Geometry check sheet. Reference: the model listing, model coordinates, mm. A direction names the side the tool comes from. Coordinates: 2 decimals unless noted, no trailing zeros. Write each loop counter-clockwise with the first axis right and the second up, starting at its lowest first coordinate (ties: lowest second). Pieces come first, ordered by that corner, then holes. Notation, with made-up numbers: (32.5, -10.5) -> (67.5, -10.5) arc R13 cw to (67.5, -4.5) -> close; hole circle Ø1 at (-26, -0.5). An arc over 180 degrees is marked (long way). Use a Markdown table: item, result.
```python
from build123d import *

# Parameters (mm, degrees)
SKETCH1_R           = 1.5
BOSS_EXTRUDE1_DEPTH = 25
SKETCH2_R           = 20
CUT_EXTRUDE1_DEPTH  = 23
CUT_EXTRUDE2_START  = -20
SKETCH3_R           = 1.5
CUT_EXTRUDE2_DEPTH  = 20
FILLET2_R           = 3
SKETCH4_R           = 22.5
SKETCH4_R_2         = 20
CUT_EXTRUDE3_DEPTH  = 2
CUT_EXTRUDE4_START  = -15
SKETCH5_R           = 24
CUT_EXTRUDE4_DEPTH  = 15
SKETCH6_R           = 22
CUT_EXTRUDE5_DEPTH  = 5


with BuildPart() as part:
    # Sketch1 → Boss-Extrude1 (new body)
    with BuildSketch(Plane(origin=(0, 0, 0), x_dir=(1, 0, 0), z_dir=(0, 1, 0))):
        with BuildLine():
            Line((13.169048105, 24), (-13.169048105, 24))
            Line((-13.169048105, 24), (-23.169048105, 26.882623622))
            ThreePointArc((-23.169048105, 26.882623622), (-26.121320344, 26.121320344), (-26.882623622, 23.169048105))
            Line((-26.882623622, 23.169048105), (-24, 13.169048105))
            Line((-24, 13.169048105), (-24, -13.169048105))
            Line((-24, -13.169048105), (-26.882623622, -23.169048105))
            ThreePointArc((-26.882623622, -23.169048105), (-26.121320344, -26.121320344), (-23.169048105, -26.882623622))
            Line((-23.169048105, -26.882623622), (-13.169048105, -24))
            Line((-13.169048105, -24), (13.169048105, -24))
            Line((13.169048105, -24), (23.169048105, -26.882623622))
            ThreePointArc((23.169048105, -26.882623622), (26.121320344, -26.121320344), (26.882623622, -23.169048105))
            Line((26.882623622, -23.169048105), (24, -13.169048105))
            Line((24, -13.169048105), (24, 13.169048105))
            Line((24, 13.169048105), (26.882623622, 23.169048105))
            ThreePointArc((26.882623622, 23.169048105), (26.121320344, 26.121320344), (23.169048105, 26.882623622))
            Line((23.169048105, 26.882623622), (13.169048105, 24))
        make_face()
        with Locations(Location((24, 24, 0), (0, 0, 270))):
            Circle(SKETCH1_R, mode=Mode.SUBTRACT)
        with Locations(Location((-24, -24, 0), (0, 0, 270))):
            Circle(SKETCH1_R, mode=Mode.SUBTRACT)
        with Locations(Location((24, -24, 0), (0, 0, 270))):
            Circle(SKETCH1_R, mode=Mode.SUBTRACT)
        with Locations(Location((-24, 24, 0), (0, 0, 270))):
            Circle(SKETCH1_R, mode=Mode.SUBTRACT)
    extrude(amount=BOSS_EXTRUDE1_DEPTH)

    # Sketch2 → Cut-Extrude1 (cut)
    with BuildSketch(Plane.XZ):
        with Locations(Location((0, 0, 0), (0, 0, 270))):
            Circle(SKETCH2_R)
    extrude(amount=-CUT_EXTRUDE1_DEPTH, mode=Mode.SUBTRACT)

    # Sketch3 → Cut-Extrude2 (cut)
    # profile 1 of 4: a face of its own
    with BuildSketch(Plane(origin=(0, 25, 0), x_dir=(1, 0, 0), z_dir=(0, 1, 0)).offset(CUT_EXTRUDE2_START)):
        with BuildLine():
            ThreePointArc((-24, 0), (-16.970562748, 16.970562748), (0, 24))
            Line((0, 24), (-13.169048105, 24))
            Line((-13.169048105, 24), (-23.169048105, 26.882623622))
            ThreePointArc((-23.169048105, 26.882623622), (-26.121320344, 26.121320344), (-26.882623622, 23.169048105))
            Line((-26.882623622, 23.169048105), (-24, 13.169048105))
            Line((-24, 13.169048105), (-24, 0))
        make_face()
        with Locations(Location((-24, 24, 0), (0, 0, 270))):
            Circle(SKETCH3_R, mode=Mode.SUBTRACT)
    # profile 2 of 4: a face of its own
    with BuildSketch(Plane(origin=(0, 25, 0), x_dir=(1, 0, 0), z_dir=(0, 1, 0)).offset(CUT_EXTRUDE2_START)):
        with BuildLine():
            Line((-13.169048105, -24), (0, -24))
            ThreePointArc((0, -24), (-16.970562748, -16.970562748), (-24, 0))
            Line((-24, 0), (-24, -13.169048105))
            Line((-24, -13.169048105), (-26.882623622, -23.169048105))
            ThreePointArc((-26.882623622, -23.169048105), (-26.121320344, -26.121320344), (-23.169048105, -26.882623622))
            Line((-23.169048105, -26.882623622), (-13.169048105, -24))
        make_face()
        with Locations(Location((-24, -24, 0), (0, 0, 270))):
            Circle(SKETCH3_R, mode=Mode.SUBTRACT)
    # profile 3 of 4: a face of its own
    with BuildSketch(Plane(origin=(0, 25, 0), x_dir=(1, 0, 0), z_dir=(0, 1, 0)).offset(CUT_EXTRUDE2_START)):
        with BuildLine():
            Line((24, -13.169048105), (24, 0))
            ThreePointArc((24, 0), (16.970562748, -16.970562748), (0, -24))
            Line((0, -24), (13.169048105, -24))
            Line((13.169048105, -24), (23.169048105, -26.882623622))
            ThreePointArc((23.169048105, -26.882623622), (26.121320344, -26.121320344), (26.882623622, -23.169048105))
            Line((26.882623622, -23.169048105), (24, -13.169048105))
        make_face()
        with Locations(Location((24, -24, 0), (0, 0, 270))):
            Circle(SKETCH3_R, mode=Mode.SUBTRACT)
    # profile 4 of 4: a face of its own
    with BuildSketch(Plane(origin=(0, 25, 0), x_dir=(1, 0, 0), z_dir=(0, 1, 0)).offset(CUT_EXTRUDE2_START)):
        with BuildLine():
            Line((24, 0), (24, 13.169048105))
            Line((24, 13.169048105), (26.882623622, 23.169048105))
            ThreePointArc((26.882623622, 23.169048105), (26.121320344, 26.121320344), (23.169048105, 26.882623622))
            Line((23.169048105, 26.882623622), (13.169048105, 24))
            Line((13.169048105, 24), (0, 24))
            ThreePointArc((0, 24), (16.970562748, 16.970562748), (24, 0))
        make_face()
        with Locations(Location((24, 24, 0), (0, 0, 270))):
            Circle(SKETCH3_R, mode=Mode.SUBTRACT)
    extrude(amount=CUT_EXTRUDE2_DEPTH, mode=Mode.SUBTRACT)

    # Fillet2
    fillet2_edges = [part.edges().sort_by_distance(p)[0] for p in [
        (0, 23, 20),
    ]]
    fillet(fillet2_edges, radius=FILLET2_R)

    # Sketch4 → Cut-Extrude3 (cut)
    with BuildSketch(Plane.XZ):
        with Locations(Location((0, 0, 0), (0, 0, 270))):
            Circle(SKETCH4_R)
        with Locations(Location((0, 0, 0), (0, 0, 270))):
            Circle(SKETCH4_R_2, mode=Mode.SUBTRACT)
    extrude(amount=-CUT_EXTRUDE3_DEPTH, mode=Mode.SUBTRACT)

    # Sketch5 → Cut-Extrude4 (cut)
    with BuildSketch(Plane(origin=(0, 25, 0), x_dir=(1, 0, 0), z_dir=(0, 1, 0)).offset(CUT_EXTRUDE4_START)):
        with Locations(Location((0, 0, 0), (0, 0, 270))):
            Circle(SKETCH5_R)
    extrude(amount=CUT_EXTRUDE4_DEPTH, mode=Mode.SUBTRACT)

    # Sketch6 → Cut-Extrude5 (cut)
    with BuildSketch(Plane(origin=(0, 10, 0), x_dir=(1, 0, 0), z_dir=(0, 1, 0))):
        with Locations(Location((0, 0, 0), (0, 0, 270))):
            Circle(SKETCH6_R)
    extrude(amount=-CUT_EXTRUDE5_DEPTH, mode=Mode.SUBTRACT)


solid = part.part
```
Item 1: Tool access check on faces 1 (the flat face through (19, 5, -20)), 2 (the flat face through (25.46, 2.46, 18.24)), 3 (the flat face through (-25.42, 2.46, 18.1)), 4 (the flat face through (-18, 5, 10)), 5 (the flat face through (19, 5, 20)). Record the directions out of +Z, -Z, +X, -X, +Y, -Y that give a thin tool (end or side, any length) a straight path to the whole face; none if there is none.
Answer block:
| item | result |
|---|---|
| face 1 | -Z, +X, +Y |
| face 2 | +X, +Y, -Y |
| face 3 | -X, +Y, -Y |
| face 4 | +Y |
| face 5 | +Z, +X, +Y |
Item 2: Section check A-A on y = 3.75. Record the boundary of the cut face in (x, z), then the cut area to 3 significant figures.
Answer block:
| item | result |
|---|---|
| outline | (-26.88, -23.17) arc R3 ccw to (-23.17, -26.88) -> (-13.17, -24) -> (13.17, -24) -> (23.17, -26.88) arc R3 ccw to (26.88, -23.17) -> (24, -13.17) -> (24, 13.17) -> (26.88, 23.17) arc R3 ccw to (23.17, 26.88) -> (13.17, 24) -> (-13.17, 24) -> (-23.17, 26.88) arc R3 ccw to (-26.88, 23.17) -> (-24, 13.17) -> (-24, -13.17) -> close; hole circle Ø3 at (-24, -24); hole circle Ø3 at (-24, 24); hole circle Ø40 at (0, 0); hole circle Ø3 at (24, -24); hole circle Ø3 at (24, 24) |
| area | 1,180 mm^2 |
Item 3: Section check D-D on y = 8.5. Record the boundary of the cut face in (x, z), then the cut area to 3 significant figures.
Answer block:
| item | result |
|---|---|
| outline | circle Ø48 at (0, 0); hole circle Ø44 at (0, 0) |
| area | 289 mm^2 |
Item 4: Thickness scan on L1, parallel to X at y = 1.5, z = 0; L2, parallel to Z at x = -6, y = 3.75; L3, parallel to Z at x = 3, y = 6.25. Record the ranges inside material, lowest first. Write a range as [from, to].
Answer block:
| item | result |
|---|---|
| L1 | x = [-24, -22.5], [22.5, 24] |
| L2 | z = [-24, -19.08], [19.08, 24] |
| L3 | z = [-23.81, -21.79], [21.79, 23.81] |
Item 5: Depth check by flat-ended pin: P1, Ø4, axis at x = 6, y = 1.5, coming from the -Z side; P2, Ø1.5, axis at x = -2, y = 2, coming from the +Z side; P3, Ø5, axis at x = -11.5, y = 1, coming from the +Z side. Enter the tip coordinate at first touch or a pass-through.
Answer block:
| item | result |
|---|---|
| P1 | stops at z = -24 |
| P2 | stops at z = 24 |
| P3 | stops at z = 24.24 |
Item 6: Section check B-B on z = -10. Record the boundary of the cut face in (x, y), then the cut area to 3 significant figures.
Answer block:
| item | result |
|---|---|
| outline | (-24, 0) -> (-20.16, 0) -> (-20.16, 2) -> (-17.32, 2) -> (-17.32, 5) -> (-19.6, 5) -> (-19.6, 10) -> (-21.82, 10) -> (-21.82, 5) -> (-24, 5) -> close; (17.32, 2) -> (20.16, 2) -> (20.16, 0) -> (24, 0) -> (24, 5) -> (21.82, 5) -> (21.82, 10) -> (19.6, 10) -> (19.6, 5) -> (17.32, 5) -> close |
| area | 77.7 mm^2 |
Item 7: Mould release check, pull along Z, two halves, no side actions. Record for faces 6 (the flat face through (25.42, 2.46, -18.1)), 7 (the flat face through (-20, 5, 20)), 8 (the flat face through (18.24, 2.46, -25.46)): +Z half, -Z half, draft (parallel to the pull), parting line (faces both ways), or undercut.
Answer block:
| item | result |
|---|---|
| face 6 | undercut |
| face 7 | draft |
| face 8 | -Z half |
Item 8: Section check C-C on x = -19. Record the boundary of the cut face in (y, z) (3 decimals), then the cut area to 3 significant figures.
Answer block:
| item | result |
|---|---|
| outline | (0, -25.681) -> (5, -25.681) -> (5, -14.663) -> (10, -14.663) -> (10, -11.091) -> (5, -11.091) -> (5, -6.245) -> (2, -6.245) -> (2, -12.052) -> (0, -12.052) -> close; (0, 12.052) -> (2, 12.052) -> (2, 6.245) -> (5, 6.245) -> (5, 11.091) -> (10, 11.091) -> (10, 14.663) -> (5, 14.663) -> (5, 25.681) -> (0, 25.681) -> close |
| area | 207 mm^2 |
